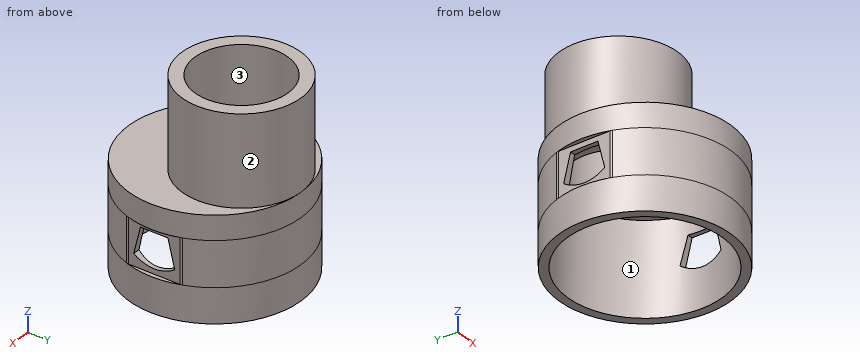
```python
from build123d import *

# Parameters (mm, degrees)
FACE005_R        = 13.5
EXTRUDE006_DEPTH = 30
FACE003_R        = 25
EXTRUDE004_DEPTH = 3
EXTRUDE003_DEPTH = 47.5
OFFSET001_R      = 25
OFFSET001_R_2    = 22.5
EXTRUDE002_DEPTH = 4
FACE_R           = 25
FACE_R_2         = 22.5
EXTRUDE_DEPTH    = 10
OFFSET_R         = 22.5
EXTRUDE001_DEPTH = 13
FILLET_R         = 2
FILLET001_R      = 2
FILLET002_R      = 2
FILLET003_R      = 2
SKETCH004_R      = 17.25
EXTRUDE005_DEPTH = 26


with BuildPart() as extrude006:
    # Face005 → Extrude006 (new body)
    with BuildSketch(Plane(origin=(0, 7.75, 56), x_dir=(0, 1, 0), z_dir=(0, 0, 1))):
        Circle(FACE005_R)
    extrude(amount=-EXTRUDE006_DEPTH)


with BuildPart() as extrude004:
    # Face003 → Extrude004 (new body)
    with BuildSketch(Plane(origin=(0, 0, 27), x_dir=(0, 1, 0), z_dir=(0, 0, 1))):
        Circle(FACE003_R)
    extrude(amount=EXTRUDE004_DEPTH)


with BuildPart() as extrude003:
    # Face002 → Extrude003 (new body)
    with BuildSketch(Plane(origin=(23.749999, 0, 16.462815), x_dir=(0, -1, 0), z_dir=(1, 0, 0))):
        with BuildLine():
            Line((-4, -5.037185), (4, -5.037185))
            Line((4, -5.037185), (6, 2.962815))
            ThreePointArc((6, 2.962815), (0, 4.962815), (-6, 2.962815))
            Line((-6, 2.962815), (-4, -5.037185))
        make_face()
    extrude(amount=-EXTRUDE003_DEPTH)


with BuildPart() as extrude002:
    # Offset001 → Extrude002 (new body)
    with BuildSketch(Plane(origin=(0, 0, 23), x_dir=(0, 1, 0), z_dir=(0, 0, 1))):
        Circle(OFFSET001_R)
        Circle(OFFSET001_R_2, mode=Mode.SUBTRACT)
    extrude(amount=EXTRUDE002_DEPTH)


with BuildPart() as fusion:
    # Face → Extrude (new body)
    with BuildSketch(Plane(origin=(0, 0, 0), x_dir=(0, 1, 0), z_dir=(0, 0, 1))):
        Circle(FACE_R)
        Circle(FACE_R_2, mode=Mode.SUBTRACT)
    extrude(amount=EXTRUDE_DEPTH)

    # Fusion: union Extrude002
    add(extrude002.part)


with BuildPart() as fusion002:
    # Offset → Extrude001 (new body)
    with BuildSketch(Plane(origin=(0, 0, 10), x_dir=(0, 1, 0), z_dir=(0, 0, 1))):
        with BuildLine():
            ThreePointArc((7.80625, -23.749999), (25, 0), (7.80625, 23.749999))
            Line((7.80625, 23.749999), (-7.80625, 23.749999))
            ThreePointArc((-7.80625, 23.749999), (-25, 0), (-7.80625, -23.749999))
            Line((-7.80625, -23.749999), (7.80625, -23.749999))
        make_face()
        Circle(OFFSET_R, mode=Mode.SUBTRACT)
    extrude(amount=EXTRUDE001_DEPTH)

    # Fillet
    fillet_edges = [fusion002.edges().sort_by_distance(p)[0] for p in [
        (23.749999, -7.80625, 16.5),
    ]]
    fillet(fillet_edges, radius=FILLET_R)

    # Fillet001
    fillet001_edges = [fusion002.edges().sort_by_distance(p)[0] for p in [
        (23.749999, 7.80625, 16.5),
    ]]
    fillet(fillet001_edges, radius=FILLET001_R)

    # Fillet002
    fillet002_edges = [fusion002.edges().sort_by_distance(p)[0] for p in [
        (-23.749999, 7.80625, 16.5),
    ]]
    fillet(fillet002_edges, radius=FILLET002_R)

    # Fillet003
    fillet003_edges = [fusion002.edges().sort_by_distance(p)[0] for p in [
        (-23.749999, -7.80625, 16.5),
    ]]
    fillet(fillet003_edges, radius=FILLET003_R)

    # Fusion001: union Fusion
    add(fusion.part)

    # Cut: cut Extrude003
    add(extrude003.part, mode=Mode.SUBTRACT)

    # Fusion002: union Extrude004
    add(extrude004.part)


with BuildPart() as cut001:
    # Sketch004 (on Face3 of Extrude004) → Extrude005 (new body)
    with BuildSketch(Plane.XY.offset(30)):
        with Locations((0, 7.75)):
            Circle(SKETCH004_R)
    extrude(amount=EXTRUDE005_DEPTH)

    # Fusion003: union Fusion002
    add(fusion002.part)

    # Cut001: cut Extrude006
    add(extrude006.part, mode=Mode.SUBTRACT)


solid = cut001.part
```
Input: part model. Units: mm. Frame: model coordinates. Face numbers are marked on the shaded views. A direction names the side the tool comes from. Coordinates: 2 decimals unless noted, no trailing zeros. Write each loop counter-clockwise with the first axis right and the second up, starting at its lowest first coordinate (ties: lowest second). Pieces come first, ordered by that corner, then holes. Notation, with made-up numbers: M -27,1.5 L 11,1.5 A28 cw 11,31.5 Z; hole C 87.25,85.25 d2. An arc over 180 degrees is marked long. Use one line per item in the form item = value.
Q1. Section A-A (y = 19). Return loops of the section in (x, z), plus the area to 3 significant figures.
Answer below:
outline = M -16.25,0 L -12.05,0 L -12.05,27 L -7.46,27 L -7.46,56 L -13.08,56 L -13.08,30 L -16.25,30 Z; M 7.46,27 L 12.05,27 L 12.05,0 L 16.25,0 L 16.25,30 L 13.08,30 L 13.08,56 L 7.46,56 Z
area = 571 mm²
Q2. Section D-D (y = 0). Count the separate pieces of the cut face and the enclosed holes in it, plus the area to 3 significant figures.
Answer below:
separate_pieces = 4
enclosed_holes = 0
area = 388 mm²
Q3. Section C-C (z = 7). Return loops of the section in (x, y).
Answer below:
outline = C 0,0 d50; hole C 0,0 d45
Q4. First-contact query: pin 1 (4 mm diameter, centred on x = 15.5, y = 7, fed in from -Z); pin 2 (6 mm diameter, centred on y = 8.5, z = 10, fed in from -X); pin 3 (10 mm diameter, centred on x = -10, z = 44.5, fed in from +Y); pin 4 (25 mm diameter, centred on x = -4.5, y = -0.5, fed in from +Z). Flat tips, straight axial feed; report the tip coordinate or a pass-through.
Answer below:
pin_1 = 27
pin_2 = -24.39
pin_3 = 24.26
pin_4 = 56
Q5. Material intervals for probe 1 along Y at (x, z) = (0, 48.25); probe 2 along X at (y, z) = (7.75, 50.25); probe 3 along Z at (x, y) = (17, 1.5), sorted ascending. Write a range as from..to.
Answer below:
probe_1 = -9.5..-5.75, 21.25..25
probe_2 = -17.25..-13.5, 13.5..17.25
probe_3 = 27..30
Q6. Set-up query: the marked faces 1, 2 and 3. Return all of +Z, -Z, +X, -X, +Y, -Y with unobstructed straight access to the full face (end or side cutting, diameter ignored); none if empty.
Answer below:
face_1 = -Z
face_2 = +Z
face_3 = +Z, -Z
Q7. Section B-B (x = -6). Return loops of the section in (y, z), plus the area to 3 significant figures.
Answer below:
outline = M -24.27,0 L -21.69,0 L -21.69,27 L -4.34,27 L -4.34,56 L -8.42,56 L -8.42,30 L -24.27,30 Z; M 19.84,27 L 21.69,27 L 21.69,0 L 24.27,0 L 24.27,30 L 23.92,30 L 23.92,56 L 19.84,56 Z
area = 425 mm²
